Design review of the part built by this model. Coordinates are the model's own, in mm. A direction names the side the tool comes from. Round coordinates to 2 decimals unless told otherwise and drop trailing zeros. Order: outer loops, then holes, each group sorted by start corner. A loop starts at its lowest first (then second) coordinate and runs counter-clockwise, first axis right, second up. Notation, with made-up numbers: M -4.5,38 L 21.5,38 A17 ccw 21.5,49 Z; hole C 52.5,80.25 d5. An arc over 180 degrees is marked long. Use a Markdown table: item, result. Add a question column.
(1) Take a section at C-C (y = 16.5). Write out the cut boundary in (x, z), then the cut area to 3 significant figures.
(2) For pin 1 (4 mm diameter, centred on x = 35, z = 42, fed in from -Y); pin 2 (3 mm diameter, centred on x = 15.5, y = 8.5, fed in from -Z), all flat-tipped, find the tip position at first contact; note any pin that passes through.
(3) Machinability: for faces 3 (the face through (17, 8, 40.25)), 4 (the face through (9.45, 18, 8)), 5 (the face through (50.45, 18, 52)), 6 (the face through (33.7, 3, 40.7)), 7 (the face through (48.115, 11.619, 28.784)), which of the approach directions +Z, -Z, +X, -X, +Y, -Y give a long, thin tool a straight path to every point of the face, cutting with its end or side? Answer none if there is none.
(4) Take a section at B-B (x = 35). Write out the cut boundary in (y, z).
(5) Take a section at A-A (z = 24). Write out the cut boundary in (x, y), then the cut area to 3 significant figures.
(6) Take a section at D-D (z = 42). Write out the cut boundary in (x, y), then the cut area to 3 significant figures.
(7) The part is to be moulded in two halves that separate along X. For faces 1 (the face through (35, 10, 0)), 2 (the face through (33.7, 3, 16.7)), say which applies: released by +X, released by -X, zero draft, split by the parting line, or undercut.
(8) To check wall thickness, follow probe 1 along X at (y, z) = (16, 45.5); probe 2 along X at (y, z) = (2.4, 30); probe 3 along Z at (x, y) = (35, 15.25). State the ranges of each line that lie inside material, in increasing order. Write a range as from..to.
```python
from build123d import *

# Parameters (mm, degrees)
SKETCH3_W           = 70
SKETCH3_H           = 60
BOSS_EXTRUDE3_DEPTH = 20
SKETCH4_R           = 1.65
CUT_EXTRUDE1_DEPTH  = 95.339811321
SKETCH6_R           = 2.1
CUT_EXTRUDE2_DEPTH  = 95.339811321
SKETCH9_R           = 3.25
CUT_EXTRUDE3_DEPTH  = 40.25
CUT_EXTRUDE4_START  = -3
SKETCH11_R          = 3
SKETCH11_R_2        = 1.65
CUT_EXTRUDE4_DEPTH  = 3
CHAMFER1_SIZE       = 0.8
CUT_EXTRUDE5_DEPTH  = 5


with BuildPart() as part:
    # Sketch3 → Boss-Extrude3 (new body)
    with BuildSketch(Plane(origin=(0, 0, 0), x_dir=(1, 0, 0), z_dir=(0, 1, 0))):
        with Locations((35, -30)):
            Rectangle(SKETCH3_W, SKETCH3_H)
    extrude(amount=BOSS_EXTRUDE3_DEPTH)

    # Sketch4 → Cut-Extrude1 (cut, through all)
    with BuildSketch(Plane(origin=(0, 20, 0), x_dir=(1, 0, 0), z_dir=(0, 1, 0))):
        with Locations(Location((35, -30, 0), (0, 0, 270))):
            Circle(SKETCH4_R)
        with Locations(Location((35, -18, 0), (0, 0, 270))):
            Circle(SKETCH4_R)
        with Locations(Location((47, -30, 0), (0, 0, 270))):
            Circle(SKETCH4_R)
        with Locations(Location((35, -42, 0), (0, 0, 270))):
            Circle(SKETCH4_R)
        with Locations(Location((23, -30, 0), (0, 0, 270))):
            Circle(SKETCH4_R)
    extrude(amount=-CUT_EXTRUDE1_DEPTH, mode=Mode.SUBTRACT)

    # Sketch6 → Cut-Extrude2 (cut, through all)
    with BuildSketch(Plane.XZ):
        with Locations(Location((61, 24, 0), (0, 0, 270))):
            Circle(SKETCH6_R)
        with Locations(Location((29, 24, 0), (0, 0, 270))):
            Circle(SKETCH6_R)
    extrude(amount=-CUT_EXTRUDE2_DEPTH, mode=Mode.SUBTRACT)

    # Sketch9 → Cut-Extrude3 (cut)
    with BuildSketch(Plane(origin=(0, 0, 0), x_dir=(-1, 0, 0), z_dir=(0, 0, -1))):
        with Locations((-53.2, 7.5)):
            Circle(SKETCH9_R)
        with Locations((-16.732176158, 7.5)):
            Circle(SKETCH9_R)
    extrude(amount=-CUT_EXTRUDE3_DEPTH, mode=Mode.SUBTRACT)

    # Sketch11 → Cut-Extrude4 (cut)
    # profile 1 of 10: a face of its own
    with BuildSketch(Plane.XZ.offset(CUT_EXTRUDE4_START)):
        with Locations(Location((35, 18, 0), (0, 0, 270))):
            Circle(SKETCH11_R)
        with Locations(Location((35, 18, 0), (0, 0, 90))):
            Circle(SKETCH11_R_2, mode=Mode.SUBTRACT)
    # profile 2 of 10: a face of its own
    with BuildSketch(Plane.XZ.offset(CUT_EXTRUDE4_START)):
        with Locations(Location((35, 30, 0), (0, 0, 270))):
            Circle(SKETCH11_R)
        with Locations(Location((35, 30, 0), (0, 0, 90))):
            Circle(SKETCH11_R_2, mode=Mode.SUBTRACT)
    # profile 3 of 10: a face of its own
    with BuildSketch(Plane.XZ.offset(CUT_EXTRUDE4_START)):
        with Locations(Location((47, 30, 0), (0, 0, 270))):
            Circle(SKETCH11_R)
        with Locations(Location((47, 30, 0), (0, 0, 90))):
            Circle(SKETCH11_R_2, mode=Mode.SUBTRACT)
    # profile 4 of 10: a face of its own
    with BuildSketch(Plane.XZ.offset(CUT_EXTRUDE4_START)):
        with Locations(Location((23, 30, 0), (0, 0, 270))):
            Circle(SKETCH11_R)
        with Locations(Location((23, 30, 0), (0, 0, 90))):
            Circle(SKETCH11_R_2, mode=Mode.SUBTRACT)
    # profile 5 of 10: a face of its own
    with BuildSketch(Plane.XZ.offset(CUT_EXTRUDE4_START)):
        with Locations(Location((35, 42, 0), (0, 0, 270))):
            Circle(SKETCH11_R)
        with Locations(Location((35, 42, 0), (0, 0, 90))):
            Circle(SKETCH11_R_2, mode=Mode.SUBTRACT)
    # profile 6 of 10: a face of its own
    with BuildSketch(Plane.XZ.offset(CUT_EXTRUDE4_START)):
        with Locations(Location((35, 42, 0), (0, 0, 90))):
            Circle(SKETCH11_R_2)
    # profile 7 of 10: a face of its own
    with BuildSketch(Plane.XZ.offset(CUT_EXTRUDE4_START)):
        with Locations(Location((23, 30, 0), (0, 0, 90))):
            Circle(SKETCH11_R_2)
    # profile 8 of 10: a face of its own
    with BuildSketch(Plane.XZ.offset(CUT_EXTRUDE4_START)):
        with Locations(Location((35, 30, 0), (0, 0, 90))):
            Circle(SKETCH11_R_2)
    # profile 9 of 10: a face of its own
    with BuildSketch(Plane.XZ.offset(CUT_EXTRUDE4_START)):
        with Locations(Location((47, 30, 0), (0, 0, 90))):
            Circle(SKETCH11_R_2)
    # profile 10 of 10: a face of its own
    with BuildSketch(Plane.XZ.offset(CUT_EXTRUDE4_START)):
        with Locations(Location((35, 18, 0), (0, 0, 90))):
            Circle(SKETCH11_R_2)
    extrude(amount=CUT_EXTRUDE4_DEPTH, mode=Mode.SUBTRACT)

    # Chamfer1
    chamfer1_edges = [part.edges().sort_by_distance(p)[0] for p in [
        (56.45, 7.5, 0),
        (19.982176158, 7.5, 0),
    ]]
    chamfer(chamfer1_edges, length=CHAMFER1_SIZE)

    # Sketch12 → Cut-Extrude5 (cut)
    with BuildSketch(Plane(origin=(0, 20, 0), x_dir=(1, 0, 0), z_dir=(0, 1, 0))):
        with BuildLine():
            Line((9.45, -60.104949747), (9.45, -44.5))
            ThreePointArc((9.45, -44.5), (14.5, -39.45), (19.55, -44.5))
            Line((19.55, -44.5), (19.55, -60.104949747))
            ThreePointArc((19.55, -60.104949747), (14.5, -65.154949747), (9.45, -60.104949747))
        make_face()
        with BuildLine():
            Line((60.55, -60.104949747), (60.55, -44.5))
            ThreePointArc((60.55, -44.5), (55.5, -39.45), (50.45, -44.5))
            Line((50.45, -44.5), (50.45, -60.104949747))
            ThreePointArc((50.45, -60.104949747), (55.5, -65.154949747), (60.55, -60.104949747))
        make_face()
        with BuildLine():
            Line((60.55, 0.104949747), (60.55, -15.5))
            ThreePointArc((60.55, -15.5), (55.5, -20.55), (50.45, -15.5))
            Line((50.45, -15.5), (50.45, 0.104949747))
            ThreePointArc((50.45, 0.104949747), (55.5, 5.154949747), (60.55, 0.104949747))
        make_face()
        with BuildLine():
            Line((9.45, 0.104949747), (9.45, -15.5))
            ThreePointArc((9.45, -15.5), (14.5, -20.55), (19.55, -15.5))
            Line((19.55, -15.5), (19.55, 0.104949747))
            ThreePointArc((19.55, 0.104949747), (14.5, 5.154949747), (9.45, 0.104949747))
        make_face()
    extrude(amount=-CUT_EXTRUDE5_DEPTH, mode=Mode.SUBTRACT)


solid = part.part
```
Verdict:
| question | item | result |
|---|---|---|
| 1 | outline | M 0,0 L 9.45,0 L 9.45,15.5 A5.05 cw 19.55,15.5 L 19.55,0 L 50.45,0 L 50.45,15.5 A5.05 cw 60.55,15.5 L 60.55,0 L 70,0 L 70,60 L 60.55,60 L 60.55,44.5 A5.05 cw 50.45,44.5 L 50.45,60 L 19.55,60 L 19.55,44.5 A5.05 cw 9.45,44.5 L 9.45,60 L 0,60 Z; hole C 23,30 d3.3; hole C 29,24 d4.2; hole C 35,18 d3.3; hole C 35,30 d3.3; hole C 35,42 d3.3; hole C 47,30 d3.3; hole C 61,24 d4.2 |
| 1 | area | 3,340 mm^2 |
| 2 | pin 1 | stops at y = 3 |
| 2 | pin 2 | stops at z = 40.25 |
| 3 | face 3 | -Z |
| 3 | face 4 | -Z, +Y |
| 3 | face 5 | +Z, +Y |
| 3 | face 6 | -Y |
| 3 | face 7 | +Y, -Y |
| 4 | outline | M 0,0 L 20,0 L 20,16.35 L 3,16.35 L 3,15 L 0,15 Z; M 0,21 L 3,21 L 3,19.65 L 20,19.65 L 20,28.35 L 3,28.35 L 3,27 L 0,27 Z; M 0,33 L 3,33 L 3,31.65 L 20,31.65 L 20,40.35 L 3,40.35 L 3,39 L 0,39 Z; M 0,45 L 3,45 L 3,43.65 L 20,43.65 L 20,60 L 0,60 Z |
| 5 | outline | M 0,0 L 26.9,0 L 26.9,20 L 0,20 Z; M 31.1,0 L 58.9,0 L 58.9,20 L 31.1,20 Z; M 63.1,0 L 70,0 L 70,20 L 63.1,20 Z; hole C 16.73,7.5 d6.5; hole C 53.2,7.5 d6.5 |
| 5 | area | 1,170 mm^2 |
| 6 | outline | M 0,0 L 32,0 L 32,3 L 33.35,3 L 33.35,20 L 18.89,20 L 18.89,15 L 10.11,15 L 10.11,20 L 0,20 Z; M 36.65,3 L 38,3 L 38,0 L 70,0 L 70,20 L 59.89,20 L 59.89,15 L 51.11,15 L 51.11,20 L 36.65,20 Z |
| 6 | area | 1,240 mm^2 |
| 7 | face 1 | zero draft |
| 7 | face 2 | undercut |
| 8 | probe 1 | x = 0..9.45, 19.55..50.45, 60.55..70 |
| 8 | probe 2 | x = 0..20, 26..32, 38..44, 50..70 |
| 8 | probe 3 | z = 0..16.35, 19.65..28.35, 31.65..40.35, 43.65..60 |
